Geometry check sheet. Reference: the model listing, model coordinates, mm. Face numbers are marked on the shaded views. A direction names the side the tool comes from. Coordinates: 2 decimals unless noted, no trailing zeros. Order: outer loops, then holes, each group sorted by start corner. A loop starts at its lowest first (then second) coordinate and runs counter-clockwise, first axis right, second up. Notation, with made-up numbers: (-40, -16.75) - (7, -16.75) arc R15 cw to (7, -4.75) - close; hole circle Ø10 at (82.5, 8.25). An arc over 180 degrees is marked (long way). One line per item, written item: value. Start each with the question number.
```python
from build123d import *

# Parameters (mm, degrees)
SKETCH1_R           = 2.5
SKETCH1_W           = 10
SKETCH1_H           = 10
BOSS_EXTRUDE1_DEPTH = 4


with BuildPart() as part:
    # Sketch1 → Boss-Extrude1 (new body)
    with BuildSketch(Plane.XY):
        with BuildLine():
            Line((5, 29.580398915), (5, 34.641016151))
            ThreePointArc((5, 34.641016151), (0, 35), (-5, 34.641016151))
            Line((-5, 34.641016151), (-5, 29.580398915))
            ThreePointArc((-5, 29.580398915), (-9.270509831, 28.531695489), (-13.341837268, 26.869971684))
            Line((-13.341837268, 26.869971684), (-16.316393446, 30.96409703))
            ThreePointArc((-16.316393446, 30.96409703), (-20.57248383, 28.315594803), (-24.40656339, 25.086244507))
            Line((-24.40656339, 25.086244507), (-21.432007211, 20.992119162))
            ThreePointArc((-21.432007211, 20.992119162), (-24.270509831, 17.633557569), (-26.587546171, 13.896128547))
            Line((-26.587546171, 13.896128547), (-31.40047917, 15.459945275))
            ThreePointArc((-31.40047917, 15.459945275), (-33.28697807, 10.815594803), (-34.490649114, 5.949380112))
            Line((-34.490649114, 5.949380112), (-29.677716115, 4.385563384))
            ThreePointArc((-29.677716115, 4.385563384), (-30, 0), (-29.677716115, -4.385563384))
            Line((-29.677716115, -4.385563384), (-34.490649114, -5.949380112))
            ThreePointArc((-34.490649114, -5.949380112), (-33.28697807, -10.815594803), (-31.40047917, -15.459945275))
            Line((-31.40047917, -15.459945275), (-26.587546171, -13.896128547))
            ThreePointArc((-26.587546171, -13.896128547), (-24.270509831, -17.633557569), (-21.432007211, -20.992119162))
            Line((-21.432007211, -20.992119162), (-24.40656339, -25.086244507))
            ThreePointArc((-24.40656339, -25.086244507), (-20.57248383, -28.315594803), (-16.316393446, -30.96409703))
            Line((-16.316393446, -30.96409703), (-13.341837268, -26.869971684))
            ThreePointArc((-13.341837268, -26.869971684), (-9.270509831, -28.531695489), (-5, -29.580398915))
            Line((-5, -29.580398915), (-5, -34.641016151))
            ThreePointArc((-5, -34.641016151), (0, -35), (5, -34.641016151))
            Line((5, -34.641016151), (5, -29.580398915))
            ThreePointArc((5, -29.580398915), (9.270509831, -28.531695489), (13.341837268, -26.869971684))
            Line((13.341837268, -26.869971684), (16.316393446, -30.96409703))
            ThreePointArc((16.316393446, -30.96409703), (20.57248383, -28.315594803), (24.40656339, -25.086244507))
            Line((24.40656339, -25.086244507), (21.432007211, -20.992119162))
            ThreePointArc((21.432007211, -20.992119162), (24.270509831, -17.633557569), (26.587546171, -13.896128547))
            Line((26.587546171, -13.896128547), (31.40047917, -15.459945275))
            ThreePointArc((31.40047917, -15.459945275), (33.28697807, -10.815594803), (34.490649114, -5.949380112))
            Line((34.490649114, -5.949380112), (29.677716115, -4.385563384))
            ThreePointArc((29.677716115, -4.385563384), (30, 0), (29.677716115, 4.385563384))
            Line((29.677716115, 4.385563384), (34.490649114, 5.949380112))
            ThreePointArc((34.490649114, 5.949380112), (33.28697807, 10.815594803), (31.40047917, 15.459945275))
            Line((31.40047917, 15.459945275), (26.587546171, 13.896128547))
            ThreePointArc((26.587546171, 13.896128547), (24.270509831, 17.633557569), (21.432007211, 20.992119162))
            Line((21.432007211, 20.992119162), (24.40656339, 25.086244507))
            ThreePointArc((24.40656339, 25.086244507), (20.57248383, 28.315594803), (16.316393446, 30.96409703))
            Line((16.316393446, 30.96409703), (13.341837268, 26.869971684))
            ThreePointArc((13.341837268, 26.869971684), (9.270509831, 28.531695489), (5, 29.580398915))
        make_face()
        with Locations((0, 17.5)):
            Circle(SKETCH1_R, mode=Mode.SUBTRACT)
        with Locations((15.155444566, 8.75)):
            Circle(SKETCH1_R, mode=Mode.SUBTRACT)
        with Locations((15.155444566, -8.75)):
            Circle(SKETCH1_R, mode=Mode.SUBTRACT)
        with Locations((0, -17.5)):
            Circle(SKETCH1_R, mode=Mode.SUBTRACT)
        with Locations((-15.155444566, -8.75)):
            Circle(SKETCH1_R, mode=Mode.SUBTRACT)
        with Locations((-15.155444566, 8.75)):
            Circle(SKETCH1_R, mode=Mode.SUBTRACT)
        Rectangle(SKETCH1_W, SKETCH1_H, mode=Mode.SUBTRACT)
    extrude(amount=BOSS_EXTRUDE1_DEPTH)


solid = part.part
```
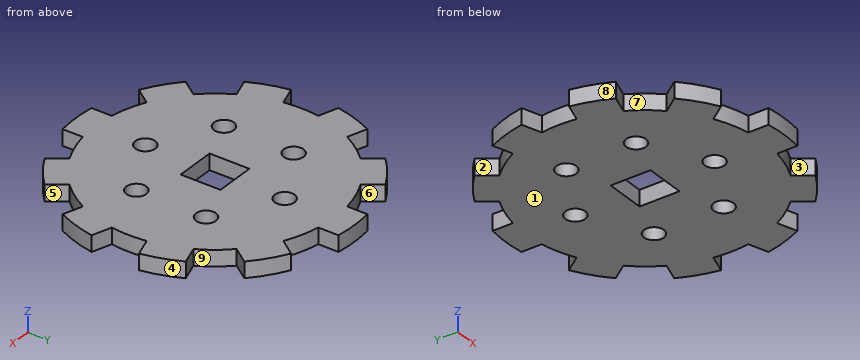
Q1. Cross-section at C-C, the plane y = -8.75. Enter the section's corners in (x, z).
Q2. Gauge pin test, flat ends, axial feed: P1, Ø1.2, axis at y = 1, z = 1, coming from the -X side; P2, Ø2, axis at y = 1.5, z = 2.5, coming from the +X side; P3, Ø1.2, axis at y = 33, z = 1.5, coming from the +X side. Record the tip position at first contact, or that the pin passes through.
Q3. Material ranges on probe 1 along Y at (x, z) = (-15.5, 3.6); probe 2 along Y at (x, z) = (-22, 0.45); probe 3 along X at (y, z) = (-3.5, 3.85), recorded low to high.
Q4. Release check for a two-part mould opening along Y. For the marked faces 6, 7, 8 and 9 record: released by +Y, released by -Y, zero draft, split by the parting line, or undercut.
Q5. Set-up check for the marked faces 1, 2, 3, 4 and 5: record each of +Z, -Z, +X, -X, +Y, -Y from which the full face is reachable in a straight line by a thin tool's end or side.
Q6. Cross-section at B-B, the plane y = 17.5. Enter the section's corners in (x, z), and give its area (3 significant figures).
Q7. Cross-section at A-A, the plane x = 0. Enter the section's corners in (y, z), and give its area (3 significant figures).
Q8. Cross-section at D-D, the plane z = 3.05. Count the separate pieces of the cut face and the enclosed holes in it, and give its area (3 significant figures).
Check result:
1. outline: (-33.89, 0) - (-17.66, 0) - (-17.66, 4) - (-33.89, 4) - close; (-12.66, 0) - (12.66, 0) - (12.66, 4) - (-12.66, 4) - close; (17.66, 0) - (33.89, 0) - (33.89, 4) - (17.66, 4) - close
2. P1: stops at x = -30
2. P2: stops at x = 30
2. P3: stops at x = 5
3. probe 1: y = -29.84 to -11.23, -6.27 to 6.27, 11.23 to 29.84
3. probe 2: y = -27.22 to -21.77, -20.4 to 20.4, 21.77 to 27.22
3. probe 3: x = -29.8 to -5, 5 to 29.8
4. face 6: released by +Y
4. face 7: undercut
4. face 8: released by -Y
4. face 9: undercut
5. face 1: -Z, +X, -X, +Y, -Y
5. face 2: +Z, -Z, -X
5. face 3: +Z, -Z, -Y
5. face 4: +Z, -Z, +X, +Y
5. face 5: +Z, -Z, +X
6. outline: (-24.37, 0) - (-2.5, 0) - (-2.5, 4) - (-24.37, 4) - close; (2.5, 0) - (24.37, 0) - (24.37, 4) - (2.5, 4) - close
6. area: 175 mm2
7. outline: (-35, 0) - (-20, 0) - (-20, 4) - (-35, 4) - close; (-15, 0) - (-5, 0) - (-5, 4) - (-15, 4) - close; (5, 0) - (15, 0) - (15, 4) - (5, 4) - close; (20, 0) - (35, 0) - (35, 4) - (20, 4) - close
7. area: 200 mm2
8. separate pieces: 1
8. enclosed holes: 7
8. area: 3,110 mm2
